```python
from build123d import *

# Parameters (mm, degrees)
BOSS_EXTRUDE1_DEPTH              = 8
BOSS_EXTRUDE2_DEPTH              = 2
SKETCH3_W                        = 22
SKETCH3_H                        = 29
CUT_EXTRUDE1_DEPTH               = 3
SKETCH4_R                        = 1.5
CUT_EXTRUDE2_DEPTH               = 5
TAP_DRILL_FOR_M3X0_5_TAP1_REACH  = 49.639
TAP_DRILL_FOR_M3X0_5_TAP1_BORE_R = 1.25
M3_CLEARANCE_HOLE1_D             = 3.4
TAP_DRILL_FOR_M3X0_5_TAP2_D      = 2.5
SKETCH10_W                       = 4
SKETCH10_H                       = 13
CUT_EXTRUDE3_DEPTH               = 2
CUT_EXTRUDE4_REACH               = 45.215


with BuildPart() as part:
    # Sketch1 → Boss-Extrude1 (new body)
    with BuildSketch(Plane(origin=(0, 0, 0), x_dir=(1, 0, 0), z_dir=(0, 1, 0))):
        with BuildLine():
            Line((-2.482050808, -4.299038106), (-3, 0))
            Line((-3, 0), (-13, 0))
            Line((-13, 0), (-13, 33))
            Line((-13, 33), (13, 33))
            Line((13, 33), (13, 0))
            Line((13, 0), (3, 0))
            Line((3, 0), (2.482050808, -4.299038106))
            ThreePointArc((2.482050808, -4.299038106), (0, -6.5), (-2.482050808, -4.299038106))
        make_face()
    extrude(amount=BOSS_EXTRUDE1_DEPTH)

    # Sketch2 → Boss-Extrude2 (add)
    with BuildSketch(Plane(origin=(0, 8, 0), x_dir=(1, 0, 0), z_dir=(0, 1, 0))):
        with BuildLine():
            Line((-11.88, 36.84), (-13, 33))
            Line((-13, 33), (-5, 33))
            Line((-5, 33), (-6.12, 36.84))
            ThreePointArc((-6.12, 36.84), (-9, 39), (-11.88, 36.84))
        make_face()
        with BuildLine():
            Line((5, 33), (13, 33))
            Line((13, 33), (11.88, 36.84))
            ThreePointArc((11.88, 36.84), (9, 39), (6.12, 36.84))
            Line((6.12, 36.84), (5, 33))
        make_face()
        with BuildLine():
            Line((-5, 0), (-13, 0))
            Line((-13, 0), (-11.88, -3.84))
            ThreePointArc((-11.88, -3.84), (-9, -6), (-6.12, -3.84))
            Line((-6.12, -3.84), (-5, 0))
        make_face()
        with BuildLine():
            Line((11.88, -3.84), (13, 0))
            Line((13, 0), (5, 0))
            Line((5, 0), (6.12, -3.84))
            ThreePointArc((6.12, -3.84), (9, -6), (11.88, -3.84))
        make_face()
    extrude(amount=-BOSS_EXTRUDE2_DEPTH)

    # Sketch3 → Cut-Extrude1 (cut)
    with BuildSketch(Plane.XZ):
        with Locations((0, -16.5)):
            Rectangle(SKETCH3_W, SKETCH3_H)
    extrude(amount=-CUT_EXTRUDE1_DEPTH, mode=Mode.SUBTRACT)

    # Sketch4 → Cut-Extrude2 (cut)
    with BuildSketch(Plane(origin=(0, 0, 0), x_dir=(-1, 0, 0), z_dir=(0, -1, 0))):
        with Locations(Location((0, -3, 0), (0, 0, 90))):
            Circle(SKETCH4_R)
    extrude(amount=-CUT_EXTRUDE2_DEPTH, mode=Mode.SUBTRACT)

    # Tap Drill for M3x0.5 Tap1 bore (on position points) → Tap Drill for M3x0.5 Tap1 (cut, up to next)
    with BuildSketch(Plane(origin=(0, 2.5, 6.5), x_dir=(1, 0, 0), z_dir=(0, 0, 1)), mode=Mode.PRIVATE) as tap_drill_for_m3x0_5_tap1_sk1:
        Circle(TAP_DRILL_FOR_M3X0_5_TAP1_BORE_R)
    tap_drill_for_m3x0_5_tap1_tool1 = extrude(tap_drill_for_m3x0_5_tap1_sk1.sketch, amount=-TAP_DRILL_FOR_M3X0_5_TAP1_REACH, mode=Mode.PRIVATE) & part.part
    add(tap_drill_for_m3x0_5_tap1_tool1.solids().sort_by_distance((0, 2.5, 6.5))[0], mode=Mode.SUBTRACT)

    # M3 Clearance Hole1 (through all)
    with Locations(Plane(origin=(0, 6, 0), x_dir=(-1, 0, 0), z_dir=(0, -1, 0))):
        with Locations((9, -3), (-9, -3), (9, 36), (-9, 36)):
            Hole(M3_CLEARANCE_HOLE1_D / 2)

    # Tap Drill for M3x0.5 Tap2 (through all)
    with Locations(Plane(origin=(0, 3, 0), x_dir=(-1, 0, 0), z_dir=(0, -1, 0))):
        with Locations((7.5, 5.5), (7.5, 27.5), (-7.5, 27.5), (-7.5, 5.5)):
            Hole(TAP_DRILL_FOR_M3X0_5_TAP2_D / 2)

    # Sketch10 → Cut-Extrude3 (cut)
    with BuildSketch(Plane(origin=(0, 3, 0), x_dir=(-1, 0, 0), z_dir=(0, -1, 0))):
        with Locations((-7, 16.5)):
            Rectangle(SKETCH10_W, SKETCH10_H)
    extrude(amount=-CUT_EXTRUDE3_DEPTH, mode=Mode.SUBTRACT)

    # Sketch19 → Cut-Extrude4 (cut, up to next)
    with BuildSketch(Plane(origin=(2.957076581, 0, 0.35626933), x_dir=(0.11961524227066314, 0, -0.992820323027551), z_dir=(0.9928203230275511, 0, 0.11961524227066316)), mode=Mode.PRIVATE) as cut_extrude4_sk1:
        with BuildLine():
            Line((-2.391154273, 0), (-2.391154273, 4))
            ThreePointArc((-2.391154273, 4), (-3.141154273, 4.75), (-3.891154273, 4))
            Line((-3.891154273, 4), (-3.891154273, 0))
            Line((-3.891154273, 0), (-2.391154273, 0))
        make_face()
    cut_extrude4_tool1 = extrude(cut_extrude4_sk1.sketch, amount=-CUT_EXTRUDE4_REACH, mode=Mode.PRIVATE) & part.part
    add(cut_extrude4_tool1.solids().sort_by_distance((2.581347, 2.297577, 3.474871))[0], mode=Mode.SUBTRACT)


solid = part.part
```
CAD build for the part. Positions are in the model's coordinates, mm. A direction names the side the tool comes from. Round coordinates to 2 decimals unless told otherwise and drop trailing zeros. Write each loop counter-clockwise with the first axis right and the second up, starting at its lowest first coordinate (ties: lowest second). Pieces come first, ordered by that corner, then holes. Notation, with made-up numbers: (58.5, -23.75) -> (105.5, -23.75) arc R16 cw to (105.5, -12.75) -> close; hole circle Ø7 at (44, -29). An arc over 180 degrees is marked (long way). Answer in a Markdown table with one row per item. Add a question column.
Item 1: Saw through at B-B, the plane y = 6.75. Count the separate pieces of the cut face and the enclosed holes in it, then the cut area to 3 significant figures.
Item 2: Saw through at D-D, the plane y = 2.5. Write the cut outline in (x, z), then the cut area to 3 significant figures.
Item 3: Drill centre lines: line 1 (X direction, y = 5.85, z = -27.5); line 2 (Z direction, x = 7.5, y = 4.6); line 3 (Z direction, x = 9, y = 7.05). Where is each one in solid material? Low to high. Write a range as from..to.
Item 4: Drop flat-ended pins along their axis: pin 1 Ø3 at (x, y) = (10, 3.5) entering from -Z; pin 2 Ø3 at (x, z) = (-7.5, -5.5) entering from -Y; pin 3 Ø1.8 at (x, z) = (-9.5, 3.5) entering from -Y; pin 4 Ø3 at (x, z) = (9.5, -35.5) entering from -Y. Give the stop position or say it passes through.
Item 5: Saw through at A-A, the plane x = 0. Write the cut outline in (y, z).
Item 6: Saw through at C-C, the plane z = -36. Write the cut outline in (x, y) (3 decimals), then the cut area to 3 significant figures.
Item 7: Which spindle directions (+Z, -Z, +X, -X, +Y, -Y) get a long thin tool onto all of the face, cutting with end or side? Do faces 4 (the face through (5.57, 7.01, -34.95)), 5 (the face through (5.55, 7.01, 1.89)), 6 (the face through (9, 6, -34)), 7 (the face through (7, 5, -17)). Say none if no direction does.
Item 8: Mould opens along X. For faces 1 (the face through (2.04, 4.75, 3.39)), 2 (the face through (12.43, 7.01, 1.95)), 3 (the face through (-9, 6, 1)) say: pulls with the +X half, pulls with the -X half, needs draft (parallel to the pull), parting line crosses it, or undercut.
Findings below:
| question | item | result |
|---|---|---|
| 1 | separate pieces | 1 |
| 1 | enclosed holes | 8 |
| 1 | area | 976 mm^2 |
| 2 | outline | (-13, -33) -> (13, -33) -> (13, 0) -> (3, 0) -> (2.67, 2.73) -> (1.44, 2.58) arc R1.5 cw (long way) to (-1.25, 3.83) -> (-1.25, 6.17) arc R2.5 ccw to (-2.48, 4.3) -> (-3, 0) -> (-13, 0) -> close; (1.25, 4.07) -> (2.49, 4.22) -> (2.48, 4.3) arc R2.5 ccw to (1.25, 6.17) -> close; hole (-11, -31) -> (11, -31) -> (11, -2) -> (-11, -2) -> close |
| 2 | area | 238 mm^2 |
| 3 | line 1 | x = -13..-8.75, -6.25..6.25, 8.75..13 |
| 3 | line 2 | z = -33..-28.75, -26.25..-23, -10..-6.75, -4.25..0 |
| 3 | line 3 | z = -39..-37.7, -34.3..1.3, 4.7..6 |
| 4 | pin 1 | stops at z = -33 |
| 4 | pin 2 | stops at y = 3 |
| 4 | pin 3 | passes through |
| 4 | pin 4 | stops at y = 6 |
| 5 | outline | (0, -33) -> (8, -33) -> (8, 6.5) -> (3.75, 6.5) -> (3.75, 4.5) -> (5, 4.5) -> (5, 1.5) -> (0, 1.5) -> (0, -2) -> (3, -2) -> (3, -31) -> (0, -31) -> close; (0, 4.5) -> (1.25, 4.5) -> (1.25, 6.5) -> (0, 6.5) -> close |
| 6 | outline | (-12.125, 6) -> (-10.7, 6) -> (-10.7, 8) -> (-12.125, 8) -> close; (-7.3, 6) -> (-5.875, 6) -> (-5.875, 8) -> (-7.3, 8) -> close; (5.875, 6) -> (7.3, 6) -> (7.3, 8) -> (5.875, 8) -> close; (10.7, 6) -> (12.125, 6) -> (12.125, 8) -> (10.7, 8) -> close |
| 6 | area | 11.4 mm^2 |
| 7 | face 4 | -Z, +Y, -Y |
| 7 | face 5 | +Z, +Y, -Y |
| 7 | face 6 | -Z, +X, -X, -Y |
| 7 | face 7 | -Y |
| 8 | face 1 | undercut |
| 8 | face 2 | pulls with the +X half |
| 8 | face 3 | needs draft |
